Check sheet for the modelled part. Datum: model origin and axes. Units: mm. A direction names the side the tool comes from. Round coordinates to 2 decimals unless told otherwise and drop trailing zeros. Order: outer loops, then holes, each group sorted by start corner. A loop starts at its lowest first (then second) coordinate and runs counter-clockwise, first axis right, second up.
Q1. Cross-section at C-C on z = 0.75. Record the cut outline in (x, y), then the cut area to 3 significant figures.
Q2. Cross-section at A-A on x = 47. Record the cut outline in (y, z) (3 decimals), then the cut area to 3 significant figures.
Q3. Cross-section at D-D on x = 35.5. Record the cut outline in (y, z).
Q4. Set-up check for faces 4 (the cylindrical face through (28.157, 8.823, 3.042)), 5 (the flat face through (47, 19, 3)), 6 (the flat face through (48.3, 32.7, 3)): record each of +Z, -Z, +X, -X, +Y, -Y from which the full face is reachable in a straight line by a thin tool's end or side.
Q5. Depth check by flat-ended pin: P1, Ø10, axis at x = 42.5, y = 7, coming from the -Z side; P2, Ø3.5, axis at x = 47, y = 12, coming from the +Z side; P3, Ø3, axis at y = 23, z = 3, coming from the +X side; P4, Ø9, axis at x = 35.5, y = 37.5, coming from the +Z side. Enter the tip coordinate at first touch or a pass-through.
Q6. Mould release check, pull along Y, two halves, no side actions. Record for faces 1 (the flat face through (50, 36, 3)), 2 (the flat face through (44, 23, 3)), 3 (the flat face through (38, 46, 3)): +Y half, -Y half, draft (parallel to the pull), parting line (faces both ways), or undercut.
Q7. Scan lines: probe 1 along Y at (x, z) = (35.5, 4.15); probe 2 along Y at (x, z) = (47, 4.75) (3 decimals); probe 3 along Y at (x, z) = (30.25, 1.1). Record each from-to range of solid material in increasing order.
Q8. Cross-section at B-B on y = 8.5. Record the cut outline in (x, z), then the cut area to 3 significant figures.
from build123d import *

# Parameters (mm, degrees)
ESQUISSE1_W             = 50
ESQUISSE1_H             = 46
BOSS_EXTRU_2_DEPTH      = 6
ESQUISSE2_W             = 27
ESQUISSE2_H             = 46
ENL_V_MAT_EXTRU_1_DEPTH = 6
ESQUISSE3_R             = 7.35
ENL_V_MAT_EXTRU_2_DEPTH = 6
ESQUISSE4_R             = 1.5
ENL_V_MAT_EXTRU_3_DEPTH = 6
ESQUISSE5_R             = 2.995
ENL_V_MAT_EXTRU_5_DEPTH = 3
ESQUISSE6_W             = 6
ESQUISSE6_H             = 8
ENL_V_MAT_EXTRU_6_DEPTH = 6


with BuildPart() as part:
    # Esquisse1 → Boss.-Extru.2 (new body)
    with BuildSketch(Plane.XY):
        with Locations((25, 23)):
            Rectangle(ESQUISSE1_W, ESQUISSE1_H)
    extrude(amount=BOSS_EXTRU_2_DEPTH)

    # Esquisse2 → Enlèv. mat.-Extru.1 (cut)
    with BuildSketch(Plane.XY.offset(6)):
        with Locations((13.5, 23)):
            Rectangle(ESQUISSE2_W, ESQUISSE2_H)
    extrude(amount=-ENL_V_MAT_EXTRU_1_DEPTH, mode=Mode.SUBTRACT)

    # Esquisse3 → Enlèv. mat.-Extru.2 (cut)
    with BuildSketch(Plane.XY.offset(6)):
        with Locations((35.5, 37.5)):
            Circle(ESQUISSE3_R)
        with Locations((35.5, 8.5)):
            Circle(ESQUISSE3_R)
    extrude(amount=-ENL_V_MAT_EXTRU_2_DEPTH, mode=Mode.SUBTRACT)

    # Esquisse4 → Enlèv. mat.-Extru.3 (cut)
    with BuildSketch(Plane.XY.offset(6)):
        with Locations((47, 34)):
            Circle(ESQUISSE4_R)
        with Locations((47, 12)):
            Circle(ESQUISSE4_R)
    extrude(amount=-ENL_V_MAT_EXTRU_3_DEPTH, mode=Mode.SUBTRACT)

    # Esquisse5 → Enlèv. mat.-Extru.5 (cut)
    with BuildSketch(Plane.XY.offset(6)):
        with Locations((47, 12)):
            Circle(ESQUISSE5_R)
        with Locations((47, 34)):
            Circle(ESQUISSE5_R)
    extrude(amount=-ENL_V_MAT_EXTRU_5_DEPTH, mode=Mode.SUBTRACT)

    # Esquisse6 → Enlèv. mat.-Extru.6 (cut)
    with BuildSketch(Plane.XY.offset(6)):
        with Locations((47, 23)):
            Rectangle(ESQUISSE6_W, ESQUISSE6_H)
    extrude(amount=-ENL_V_MAT_EXTRU_6_DEPTH, mode=Mode.SUBTRACT)


solid = part.part
Results found:
1. outline: (27, 0) - (50, 0) - (50, 19) - (44, 19) - (44, 27) - (50, 27) - (50, 46) - (27, 46) - close; hole circle Ø14.7 at (35.5, 8.5); hole circle Ø14.7 at (35.5, 37.5); hole circle Ø3 at (47, 12); hole circle Ø3 at (47, 34)
1. area: 656 mm2
2. outline: (0, 0) - (10.5, 0) - (10.5, 3) - (9.005, 3) - (9.005, 6) - (0, 6) - close; (13.5, 0) - (19, 0) - (19, 6) - (14.995, 6) - (14.995, 3) - (13.5, 3) - close; (27, 0) - (32.5, 0) - (32.5, 3) - (31.005, 3) - (31.005, 6) - (27, 6) - close; (35.5, 0) - (46, 0) - (46, 6) - (36.995, 6) - (36.995, 3) - (35.5, 3) - close
2. area: 174 mm2
3. outline: (0, 0) - (1.15, 0) - (1.15, 6) - (0, 6) - close; (15.85, 0) - (30.15, 0) - (30.15, 6) - (15.85, 6) - close; (44.85, 0) - (46, 0) - (46, 6) - (44.85, 6) - close
4. face 4: +Z, -Z
4. face 5: +Z, -Z, +X
4. face 6: +Z
5. P1: stops at z = 0
5. P2: stops at z = 3
5. P3: stops at x = 44
5. P4: passes through
6. face 1: draft
6. face 2: undercut
6. face 3: +Y half
7. probe 1: y = 0 to 1.15, 15.85 to 30.15, 44.85 to 46
7. probe 2: y = 0 to 9.005, 14.995 to 19, 27 to 31.005, 36.995 to 46
7. probe 3: y = 0 to 3.36, 13.64 to 32.36, 42.64 to 46
8. outline: (27, 0) - (28.15, 0) - (28.15, 6) - (27, 6) - close; (42.85, 0) - (50, 0) - (50, 6) - (42.85, 6) - close
8. area: 49.8 mm2
